from build123d import *

# Parameters (mm, degrees)
EXTRUDE_1_DEPTH     = 2
SKETCH_2_R          = 4.1
CUT_EXTRUDE_1_DEPTH = 10
SKETCH_3_W          = 12
SKETCH_3_H          = 1.078774048
CUT_EXTRUDE_2_DEPTH = 10


with BuildPart() as part:
    # 草图1 → 凸台-拉伸1 (new body)
    with BuildSketch(Plane.XY):
        Polygon((-6, 0), (-6, 15), (-6, 30.078774409), (6, 30.078774409), (6, 15), (6, 0), (3, 0), (3, -2), (-3, -2), (-3, 0), align=None)
    extrude(amount=EXTRUDE_1_DEPTH)

    # 草图2 → 切除-拉伸1 (cut)
    with BuildSketch(Plane.XY.offset(2)):
        with Locations((0.243619751, 8.579446227)):
            Circle(SKETCH_2_R)
    extrude(amount=-CUT_EXTRUDE_1_DEPTH, mode=Mode.SUBTRACT)

    # 草图3 → 切除-拉伸2 (cut)
    with BuildSketch(Plane.XY.offset(2)):
        with Locations((0, 29.539387385)):
            Rectangle(SKETCH_3_W, SKETCH_3_H)
        Polygon((6, 29.000000361), (10.298878861, 29.000000361), (10.298878861, 34.143483695), (-9.585000786, 34.143483695), (-9.585000786, 29.000000361), (-6, 29.000000361), (-6, 30.078774409), (6, 30.078774409), align=None)
    extrude(amount=-CUT_EXTRUDE_2_DEPTH, mode=Mode.SUBTRACT)


solid = part.part
Geometry check sheet. Reference: the model listing, model coordinates, mm. A direction names the side the tool comes from. Give positions to 0.01 mm unless a question says otherwise; leave off trailing zeros. Order: outer loops, then holes, each group sorted by start corner. A loop starts at its lowest first (then second) coordinate and runs counter-clockwise, first axis right, second up.
1. Sectioned sample at A-A (x = 0.25). Record the boundary of the cut face in (y, z).
Completed:
outline: (-2, 0) - (4.48, 0) - (4.48, 2) - (-2, 2) - close; (12.68, 0) - (29, 0) - (29, 2) - (12.68, 2) - close
2. Sectioned sample at B-B (y = 7.5). Record the boundary of the cut face in (x, z).
Completed:
outline: (-6, 0) - (-3.71, 0) - (-3.71, 2) - (-6, 2) - close; (4.2, 0) - (6, 0) - (6, 2) - (4.2, 2) - close
3. Depth check by flat-ended pin: pin 1 (1 mm diameter, centred on x = -4.5, z = 1.5, fed in from -Y). Enter the tip coordinate at first touch or a pass-through.
Completed:
pin 1: stops at y = 0
4. Scan lines: line 1 (Y direction, x = 5.75, z = 0.15); line 2 (X direction, y = 11.5, z = 1.5); line 3 (Y direction, x = 1, z = 1.1). Record each from-to range of solid material in increasing order.
Completed:
line 1: y = 0 to 29
line 2: x = -6 to -2.63, 3.12 to 6
line 3: y = -2 to 4.55, 12.61 to 29
5. Sectioned sample at D-D (x = -4.75). Record the boundary of the cut face in (y, z), then the cut area to 3 significant figures.
Completed:
outline: (0, 0) - (29, 0) - (29, 2) - (0, 2) - close
area: 58.0 mm2
6. Sectioned sample at C-C (z = 1.55). Record the boundary of the cut face in (x, y).
Completed:
outline: (-6, 0) - (-3, 0) - (-3, -2) - (3, -2) - (3, 0) - (6, 0) - (6, 29) - (-6, 29) - close; hole circle Ø8.2 at (0.24, 8.58)
7. Access from +Z, -Z, +X, -X, +Y, -Y to the whole of each face (thin tool, end or side, straight path). Record for faces 4 (the face through (5, 0, 1)), 5 (the face through (-3, -1, 1)), 6 (the face through (0, 14, 0)).
Completed:
face 4: +Z, -Z, +X, -Y
face 5: +Z, -Z, -X, -Y
face 6: -Z, +X, -X, +Y, -Y
8. Draft check along Y on faces 1 (the face through (-4, 0, 1)), 2 (the face through (0, 29, 1)), 3 (the face through (-0.29, 12.645, 1.014)). Enter one of: pulls with the +Y half, pulls with the -Y half, needs draft (parallel to the pull), parting line crosses it, or undercut.
Completed:
face 1: pulls with the -Y half
face 2: pulls with the +Y half
face 3: undercut
